from build123d import *

# Parameters (mm, degrees)
SKETCH_1_R          = 12.5
EXTRUDE_1_DEPTH     = 2
SKETCH_2_R          = 9
EXTRUDE_2_DEPTH     = 2.5
EXTRUDE_3_DEPTH     = 21.8
SKETCH_4_R          = 1.825
CUT_EXTRUDE_1_DEPTH = 32.688957067
SKETCH_5_R          = 6.25
CUT_EXTRUDE_2_DEPTH = 2


with BuildPart() as part:
    # 草图1 → 凸台-拉伸1 (new body)
    with BuildSketch(Plane.XY):
        Circle(SKETCH_1_R)
    extrude(amount=EXTRUDE_1_DEPTH)

    # 草图2 → 凸台-拉伸2 (add)
    with BuildSketch(Plane.XY.offset(2)):
        Circle(SKETCH_2_R)
    extrude(amount=EXTRUDE_2_DEPTH)

    # 草图3 → 凸台-拉伸3 (add)
    with BuildSketch(Plane.XY.offset(4.5)):
        Polygon((5.187426457, -4.595161232), (6.57323959, 2.194862476), (1.385813133, 6.790023708), (-5.187426457, 4.595161232), (-6.57323959, -2.194862476), (-1.385813133, -6.790023708), align=None)
    extrude(amount=EXTRUDE_3_DEPTH)

    # 草图4 → 切除-拉伸1 (cut, through all)
    with BuildSketch(Plane.XY.offset(26.3)):
        Circle(SKETCH_4_R)
    extrude(amount=-CUT_EXTRUDE_1_DEPTH, mode=Mode.SUBTRACT)

    # 草图5 → 切除-拉伸2 (cut)
    with BuildSketch(Plane(origin=(0, 0, 0), x_dir=(-1, 0, 0), z_dir=(0, 0, -1))):
        Circle(SKETCH_5_R)
    extrude(amount=-CUT_EXTRUDE_2_DEPTH, mode=Mode.SUBTRACT)


solid = part.part
Can you work these out from the model? Positions are in its coordinate system, mm. A direction names the side the tool comes from. Coordinates: 2 decimals unless noted, no trailing zeros. Write each loop counter-clockwise with the first axis right and the second up, starting at its lowest first coordinate (ties: lowest second). Pieces come first, ordered by that corner, then holes. Notation, with made-up numbers: (-33.5, 63.5) -> (15.5, 63.5) arc R12 cw to (15.5, 86.5) -> close; hole circle Ø3 at (-1, 62). An arc over 180 degrees is marked (long way). Write each question's results on one line, items separated by ' | '. Start each with the question number.
Q1. On a 3-axis mill with a long thin cutter (end or side, diameter ignored), from which of +Z, -Z, +X, -X, +Y, -Y can I reach the whole of each face in a straight line? I mean faces 4 (the face through (-5.87, 1.25, 15.25)), 5 (the face through (2, -6, 4.5)), 6 (the face through (4.016, 4.46, 15.247)), 7 (the face through (1.5, -1.3, 2)), 8 (the face through (5.87, -1.25, 15.25)). Say none if no direction works.
Q2. If I drill on probe 1 along Y at (x, z) = (0, 1.1); probe 2 along Z at (x, y) = (2.75, -2.75); probe 3 along Z at (x, y) = (8.5, -1.5), over which ranges is the centre line in solid material (lowest first)?
Q3. Imagine slicing it at B-B (y = 0). Write out the boundary of the cut face in (x, z) (3 decimals), then the cut area to 3 significant figures.
Q4. Imagine slicing it at A-A (z = 7.25). Write out the boundary of the cut face in (x, y) (3 decimals), then the cut area to 3 significant figures.
Q5. Imagine slicing it at C-C (x = 0.75). Write out the boundary of the cut face in (y, z).
Q6. Imagine slicing it at D-D (y = 5.5). Write out the boundary of the cut face in (x, z).
Q7. I'm going to push flat-ended pins straight in: pin 1 (3.5 mm diameter, centred on x = 0, y = 0, fed in from -Z); pin 2 (5 mm diameter, centred on x = 1, z = 16.5, fed in from -Y); pin 3 (1.5 mm diameter, centred on y = 0.5, z = 19.5, fed in from +X); pin 4 (5 mm diameter, centred on y = 9.5, z = 3, fed in from +X). Where does each tip first touch, or does it pass through?
Q8. We'd pull the mould along X, two halves only. Please class faces 1 (the face through (1.85, -5.71, 15.25)), 2 (the face through (-4.016, -4.46, 15.247)), 3 (the face through (-5.96, 1.88, 0.99)): +X half, -X half, draft (parallel to the pull), parting line (faces both ways), or undercut.
Taken from the geometry:
1) face 4: +Z, -X, +Y | face 5: +Z | face 6: +Z, +X, +Y | face 7: -Z | face 8: +Z, +X, -Y
2) probe 1: y = -12.5 to -6.25, 6.25 to 12.5 | probe 2: z = 2 to 26.3 | probe 3: z = 0 to 4.5
3) outline: (-12.5, 0) -> (-6.25, 0) -> (-6.25, 2) -> (-1.825, 2) -> (-1.825, 26.3) -> (-6.125, 26.3) -> (-6.125, 4.5) -> (-9, 4.5) -> (-9, 2) -> (-12.5, 2) -> close; (1.825, 2) -> (6.25, 2) -> (6.25, 0) -> (12.5, 0) -> (12.5, 2) -> (9, 2) -> (9, 4.5) -> (6.125, 4.5) -> (6.125, 26.3) -> (1.825, 26.3) -> close | area: 248 mm^2
4) outline: (-6.573, -2.195) -> (-1.386, -6.79) -> (5.187, -4.595) -> (6.573, 2.195) -> (1.386, 6.79) -> (-5.187, 4.595) -> close; hole circle Ø3.65 at (0, 0) | area: 114 mm^2
5) outline: (-12.48, 0) -> (-6.2, 0) -> (-6.2, 2) -> (-1.66, 2) -> (-1.66, 26.3) -> (-6.08, 26.3) -> (-6.08, 4.5) -> (-8.97, 4.5) -> (-8.97, 2) -> (-12.48, 2) -> close; (1.66, 2) -> (6.2, 2) -> (6.2, 0) -> (12.48, 0) -> (12.48, 2) -> (8.97, 2) -> (8.97, 4.5) -> (6.58, 4.5) -> (6.58, 26.3) -> (1.66, 26.3) -> close
6) outline: (-11.22, 0) -> (-2.97, 0) -> (-2.97, 2) -> (2.97, 2) -> (2.97, 0) -> (11.22, 0) -> (11.22, 2) -> (7.12, 2) -> (7.12, 4.5) -> (2.84, 4.5) -> (2.84, 26.3) -> (-2.48, 26.3) -> (-2.48, 4.5) -> (-7.12, 4.5) -> (-7.12, 2) -> (-11.22, 2) -> close
7) pin 1: passes through | pin 2: stops at y = -6.79 | pin 3: stops at x = 6.38 | pin 4: stops at x = 10.21
8) face 1: +X half | face 2: -X half | face 3: undercut
